Autodesk Inventor part; units mm, degrees
ref_plane "YZ Plane" through (0, 0, 0) normal (1, 0, 0) x (0, 1, 0)
ref_plane "XZ Plane" through (0, 0, 0) normal (0, 1, 0) x (-1, 0, 0)
ref_plane "XY Plane" through (0, 0, 0) normal (0, 0, 1) x (1, 0, 0)
sketch "main" plane through (0, 0, 0) normal (0, 0, 1) x (1, 0, 0)
  circle A0 centre (36.5381, -21.0803) radius 2.1844
  circle A1 centre (-26.9619, -21.0803) radius 2.1844
  circle A2 centre (-37.1219, 30.698) radius 2.1844
  circle A3 centre (45.8515, -1.2181) radius 2.1844
  circle A4 centre (-55.3252, 16.2075) radius 2.1844
  point P0 (-7.4039, 0.7054)
sketch "Sketch1" plane through (0, 0, 0) normal (0, 0, 1) x (1, 0, 0)
  arc A0 (-21.1694, -10.7645) -> (-21.9938, -17.3739) centre (-18.2033, -14.4906) ccw
  arc A1 (1.7098, 4.445) -> (-2.9661, 3.7261) centre (0, 0) ccw
  arc A2 (6.3695, -54.6616) -> (10.16, -56.5408) centre (10.16, -51.7783) ccw
  arc A3 (73.66, -56.5408) -> (77.972, -53.8002) centre (73.66, -51.7783) ccw
  arc A4 (87.2853, -33.938) -> (84.6831, -27.4711) centre (82.9733, -31.9161) ccw
  line L0 (77.972, -53.8002) -> (87.2853, -33.938)
  line L1 (-2.9661, 3.7261) -> (-21.1694, -10.7645)
  line L2 (-21.9938, -17.3739) -> (6.3695, -54.6616)
  line L3 (-5.9701, -14.8978) -> (-2.7997, -12.374)
  line L4 (70.5159, -39.7871) -> (69.0435, -42.9273)
  line L5 (67.6061, -43.8408) -> (44.5028, -43.8408)
  line L6 (-0.0927, -25.1889) -> (-6.2449, -17.1009)
  line L7 (-0.2827, -13.1866) -> (2.6991, -23.7983)
  line L8 (13.8548, -16.552) -> (17.9845, -31.2486)
  line L9 (35.8381, -40.6928) -> (69.3364, -38.0816)
  line L10 (19.6361, -32.4018) -> (47.9716, -30.1931)
  arc A5 (-0.2827, -13.1866) -> (-2.7997, -12.374) centre (-1.811, -13.6161) ccw
  arc A6 (-5.9701, -14.8978) -> (-6.2449, -17.1009) centre (-4.9814, -16.1398) ccw
  arc A7 (-0.0927, -25.1889) -> (2.6991, -23.7983) centre (1.1708, -24.2278) ccw
  arc A8 (15.9531, -14.6409) -> (13.8548, -16.552) centre (15.3831, -16.1225) ccw
  arc A9 (17.9845, -31.2486) -> (19.6361, -32.4018) centre (19.5128, -30.8191) ccw
  arc A10 (47.9716, -30.1931) -> (48.4182, -27.1287) centre (47.8482, -28.6104) ccw
  arc A11 (67.6061, -43.8408) -> (69.0435, -42.9273) centre (67.6061, -42.2533) ccw
  arc A12 (70.5159, -39.7871) -> (69.3364, -38.0816) centre (69.4296, -39.2778) ccw
  circle A13 centre (35.56, -51.7783) radius 5.5563
  line L11 (10.16, -56.5408) -> (27.7829, -56.5408)
  line L12 (43.3371, -56.5408) -> (73.66, -56.5408)
  arc A14 (30.0049, -57.448) -> (41.1151, -57.448) centre (35.56, -51.7783) ccw
  arc A15 (42.5123, -43.1393) -> (35.8381, -40.6928) centre (35.56, -51.7783) ccw
  arc A16 (30.0049, -57.448) -> (27.7829, -56.5408) centre (27.7829, -59.7158) ccw
  arc A17 (43.3371, -56.5408) -> (41.1151, -57.448) centre (43.3371, -59.7158) ccw
  arc A18 (42.5123, -43.1393) -> (44.5028, -43.8408) centre (44.5028, -40.6658) ccw
  circle A19 centre (35.56, -13.6783) radius 5.5563
  line L13 (1.7098, 4.445) -> (31.3431, -6.9536)
  line L14 (43.1965, -11.513) -> (84.6831, -27.4711)
  arc A20 (32.7104, -21.0867) -> (32.7104, -21.0867) centre (35.56, -13.6783) ccw
  arc A21 (43.1965, -11.513) -> (31.3431, -6.9536) centre (35.56, -13.6783) ccw
  line L15 (15.9531, -14.6409) -> (32.7104, -21.0867)
  line L16 (32.7104, -21.0867) -> (48.4182, -27.1287)
  circle A22 centre (73.66, -51.7783) radius 2.1844
  circle A23 centre (10.16, -51.7783) radius 2.1844
  circle A24 centre (0, 0) radius 2.1844
  circle A25 centre (82.9733, -31.9161) radius 2.1844
  circle A26 centre (-18.2033, -14.4906) radius 2.1844
  point P0 (0, 0)
  point P1 (17.1709, -28.3531)
  point P2 (29.21, -56.5408)
  point P3 (41.91, -56.5408)
  point P4 (43.3035, -43.8408)
  dimension "d0" = 9.525
  dimension "d1" = 9.525
  dimension "d2" = 9.525
  dimension "d3" = 9.525
  dimension "d4" = 9.525
  dimension "d5" = 12.7
  dimension "d7" = 9.525
  dimension "d8" = 1.5875
  dimension "d9" = 1.5875
  dimension "d13" = 11.1125
  dimension "d16" = 3.175
  dimension "d18" = 11.1125
  dimension "d20" = 12.7
  dimension "d21" = 12.7
  dimension "d22" = 12.7
  dimension "d23" = 12.7
extrude "Extrusion1" add sketch "Sketch1" along normal blind 1.5875
properties part number "gearbox_gusset" material "Acetal Resin, White"
Check sheet for the modelled part. Datum: model origin and axes. Units: mm. A direction names the side the tool comes from. Round coordinates to 2 decimals unless told otherwise and drop trailing zeros. Order: outer loops, then holes, each group sorted by start corner. A loop starts at its lowest first (then second) coordinate and runs counter-clockwise, first axis right, second up.
(1) Go/stop test with flat-tipped pins: P1, Ø6, axis at x = 36, y = -45.5, coming from the -Z side; P2, Ø0.5, axis at x = 53, z = 1, coming from the +Y side. Record where each tip stops, or that it passes through.
(2) Cross-section at B-B, the plane x = 46. Enter the section's corners in (y, z), and give its area (3 significant figures).
(3) Draft check along X on faces 1 (the cylindrical face through (39.33, -41.35, 0.78)), 2 (the flat face through (63.65, -19.38, 0.78)), 3 (the flat face through (32, -34, 1.588)). Enter one of: pulls with the +X half, pulls with the -X half, needs draft (parallel to the pull), parting line crosses it, or undercut.
(4) Scan lines: probe 1 along Y at (x, z) = (46.5, 0.4); probe 2 along X at (y, z) = (-55, 0.5); probe 3 along Y at (x, z) = (73.66, 1.2). Record each from-to range of solid material in increasing order.
(5) Cross-section at A-A, the plane y = 0. Enter the section's corners in (x, z), and give its area (3 significant figures).
(6) Access from +Z, -Z, +X, -X, +Y, -Y to the whole of each face (thin tool, end or side, straight path). Record for faces 4 (the flat face through (-4.407, -13.654, 0.783)), 5 (the flat face through (32, -34, 0)).
(7) Cross-section at C-C, the plane z = 0.6. State how many separate pieces and enclosed holes the cut face has, and give its area (3 significant figures).
Check sheet entries:
1. P1: stops at z = 0
1. P2: stops at y = -15.19
2. outline: (-56.54, 0) - (-43.84, 0) - (-43.84, 1.59) - (-56.54, 1.59) - close; (-39.9, 0) - (-30.35, 0) - (-30.35, 1.59) - (-39.9, 1.59) - close; (-26.2, 0) - (-12.59, 0) - (-12.59, 1.59) - (-26.2, 1.59) - close
2. area: 56.9 mm2
3. face 1: undercut
3. face 2: pulls with the +X half
3. face 3: needs draft
4. probe 1: y = -56.54 to -43.84, -39.86 to -30.31, -26.39 to -12.78
4. probe 2: x = 6.65 to 31.03, 40.09 to 77.17
4. probe 3: y = -56.54 to -53.96, -49.59 to -23.23
5. outline: (-7.65, 0) - (-2.18, 0) - (-2.18, 1.59) - (-7.65, 1.59) - close; (2.18, 0) - (13.27, 0) - (13.27, 1.59) - (2.18, 1.59) - close
5. area: 26.3 mm2
6. face 4: +Z, -Z
6. face 5: -Z, +X, -X, +Y, -Y
7. separate pieces: 1
7. enclosed holes: 10
7. area: 3,640 mm2
